```python
from build123d import *

# Parameters (mm, degrees)
SKETCH1_R                                           = 133.35
EXTRUDE_CENTER_HOLE_DEPTH                           = 6.35
CSK_FOR_1_4_FLAT_HEAD_MACHINE_SCREW_100_D           = 6.7564
CSK_FOR_1_4_FLAT_HEAD_MACHINE_SCREW_100_CSINK_D     = 12.8778
CSK_FOR_1_4_FLAT_HEAD_MACHINE_SCREW_100_CSINK_ANGLE = 100


with BuildPart() as part:
    # Sketch1 → Extrude & center hole (new body)
    with BuildSketch(Plane(origin=(0, 0, 0), x_dir=(1, 0, 0), z_dir=(0, 1, 0))):
        Polygon((0, 171.45), (146.05, 171.45), (146.05, 0), (146.05, -171.45), (-146.05, -171.45), (-146.05, 0), (-146.05, 171.45), align=None)
        Circle(SKETCH1_R, mode=Mode.SUBTRACT)
    extrude(amount=EXTRUDE_CENTER_HOLE_DEPTH)

    # CSK for 1/4 Flat Head Machine Screw (100)1 (through all)
    with Locations(Plane(origin=(0, 6.35, 0), x_dir=(1, 0, 0), z_dir=(0, 1, 0))):
        with Locations((-114.3, -158.75), (114.3, -158.75), (127, 158.75), (-127, 158.75)):
            CounterSinkHole(CSK_FOR_1_4_FLAT_HEAD_MACHINE_SCREW_100_D / 2, CSK_FOR_1_4_FLAT_HEAD_MACHINE_SCREW_100_CSINK_D / 2, counter_sink_angle=CSK_FOR_1_4_FLAT_HEAD_MACHINE_SCREW_100_CSINK_ANGLE)


solid = part.part
```
For this review, take the finished solid that the model builds, in its own axes (mm). Coordinates: 2 decimals unless noted, no trailing zeros. Write each loop counter-clockwise with the first axis right and the second up, starting at its lowest first coordinate (ties: lowest second). Pieces come first, ordered by that corner, then holes.
(1) Wall thickness on probe 1 along X at (y, z) = (2, -158.75); probe 2 along X at (y, z) = (1.55, 158.75); probe 3 along Z at (x, y) = (-113, 6.25): over which ranges is each line inside the solid? List them lowest first.
(2) Add section A-A on x = 0. Give the boundary of the cut face in (y, z).
(3) Add section B-B on y = 1.75. Give the boundary of the cut face in (x, z), then the cut area to 3 significant figures.
(4) The part is to be moulded in two halves that separate along X. For faces 1 (the face through (-113.84, 3.91, 155.25)), 2 (the face through (67, 0, -117)), say which applies: +X half, -X half, draft (parallel to the pull), parting line (faces both ways), or undercut.
(5) For pin 1 Ø8 at (x, z) = (127, -158.75) entering from -Y; pin 2 Ø8 at (x, z) = (-127, -158.75) entering from +Y, all flat-tipped, find the tip position at first contact; note any pin that passes through.
(6) Add section C-C on z = 0. Give the boundary of the cut face in (x, y), then the cut area to 3 significant figures.
Answer sheet:
1. probe 1: x = -146.05 to -130.38, -123.62 to 123.62, 130.38 to 146.05
1. probe 2: x = -146.05 to -117.68, -110.92 to 110.92, 117.68 to 146.05
1. probe 3: z = -171.45 to -70.8, 70.8 to 152.57, 164.93 to 171.45
2. outline: (0, -171.45) - (6.35, -171.45) - (6.35, -133.35) - (0, -133.35) - close; (0, 133.35) - (6.35, 133.35) - (6.35, 171.45) - (0, 171.45) - close
3. outline: (-146.05, -171.45) - (146.05, -171.45) - (146.05, 171.45) - (-146.05, 171.45) - close; hole circle Ø266.7 at (0, 0); hole circle Ø6.76 at (-127, -158.75); hole circle Ø6.76 at (-114.3, 158.75); hole circle Ø6.76 at (114.3, 158.75); hole circle Ø6.76 at (127, -158.75)
3. area: 44,200 mm2
4. face 1: undercut
4. face 2: draft
5. pin 1: stops at y = 0
5. pin 2: stops at y = 4.3
6. outline: (-146.05, 0) - (-133.35, 0) - (-133.35, 6.35) - (-146.05, 6.35) - close; (133.35, 0) - (146.05, 0) - (146.05, 6.35) - (133.35, 6.35) - close
6. area: 161 mm2
